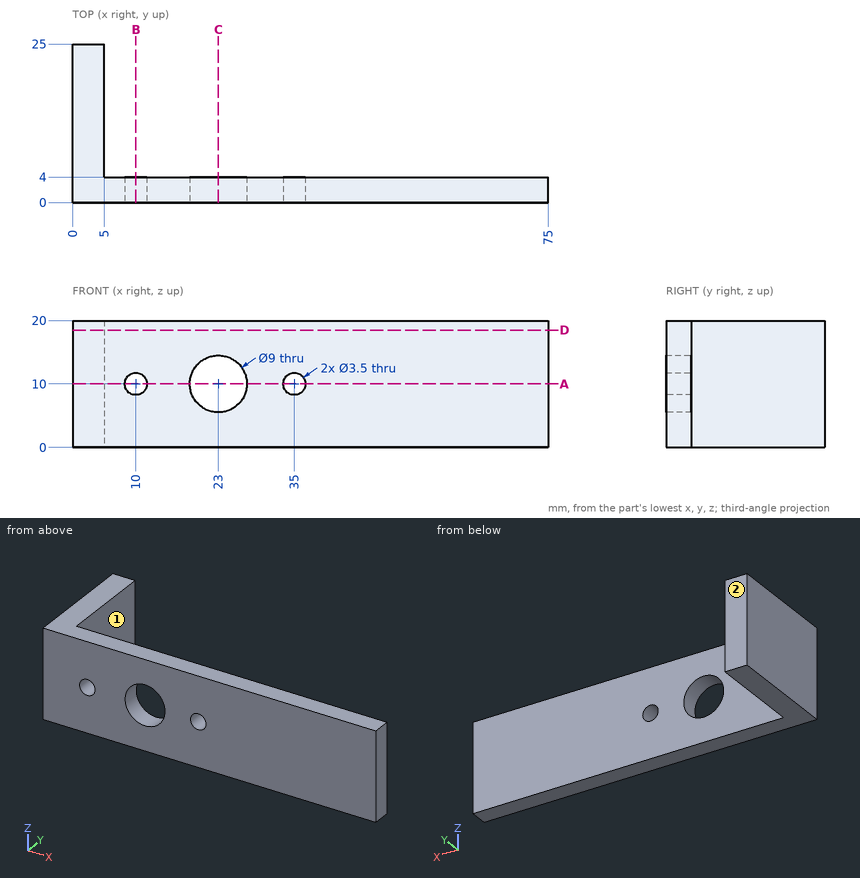
Answer from the drawing. Dimensions are ordinates in mm from the lowest x, y and z of the part. A direction names the side the tool comes from. Give positions to 0.01 mm unless a question says otherwise; leave off trailing zeros. Loops run counter-clockwise (first coordinate to the right, second up) from the corner with the lowest first, then second, coordinate; pieces in that order, holes last.
Item 1: A tool of negligible diameter and unlimited length cuts with its end or side. For the marked faces 1 and 2, from which of +Z, -Z, +X, -X, +Y, -Y can it reach the whole face along a straight path? Write none if from no direction.
Derived:
face 1: +Z, -Z, +X, +Y
face 2: +Z, -Z, +X, -X, +Y
Item 2: A cutting plane is placed at D-D (z = 18.5). Give the vertices of the cut face in (x, y).
Derived:
outline: (0, 0) - (75, 0) - (75, 4) - (5, 4) - (5, 25) - (0, 25) - close
Item 3: A cutting plane is placed at B-B (x = 10). Give the vertices of the cut face in (y, z).
Derived:
outline: (0, 0) - (4, 0) - (4, 8.25) - (0, 8.25) - close; (0, 11.75) - (4, 11.75) - (4, 20) - (0, 20) - close
Item 4: Find the intervals of material crossed by line 1 along X through (y, z) = (2.8, 10); line 2 along X through (y, z) = (16.5, 11.5); line 3 along Y through (x, z) = (22, 1.25), in increasing order.
Derived:
line 1: x = 0 to 8.25, 11.75 to 18.5, 27.5 to 33.25, 36.75 to 75
line 2: x = 0 to 5
line 3: y = 0 to 4
Item 5: A cutting plane is placed at C-C (x = 23). Give the vertices of the cut face in (y, z), then the cut area to 3 significant figures.
Derived:
outline: (0, 0) - (4, 0) - (4, 5.5) - (0, 5.5) - close; (0, 14.5) - (4, 14.5) - (4, 20) - (0, 20) - close
area: 44.0 mm2
Item 6: This flat-tipped pin is pushed along its axis until it touches: pin 1 Ø6 at (x, z) = (24.5, 6) entering from +Y. Where does it stop, or does it pass through?
Derived:
pin 1: stops at y = 4
Item 7: A cutting plane is placed at A-A (z = 10). Give the vertices of the cut face in (x, y), then the cut area to 3 significant figures.
Derived:
outline: (0, 0) - (8.25, 0) - (8.25, 4) - (5, 4) - (5, 25) - (0, 25) - close; (11.75, 0) - (18.5, 0) - (18.5, 4) - (11.75, 4) - close; (27.5, 0) - (33.25, 0) - (33.25, 4) - (27.5, 4) - close; (36.75, 0) - (75, 0) - (75, 4) - (36.75, 4) - close
area: 341 mm2
